Autodesk Inventor part; units mm, degrees
ref_plane "Work Plane1" through (29, 0, 0) normal (0, -1, 0) x (1, 0, 0)
ref_plane "YZ Plane" through (0, 0, 0) normal (1, 0, 0) x (0, 1, 0)
ref_plane "XZ Plane" through (0, 0, 0) normal (0, 1, 0) x (-1, 0, 0)
sketch "Sketch1" plane through (0, 0, 0) normal (0, 0, 1) x (1, 0, 0)
  line L0 (-1, 0) -> (16, 0)
  line L1 (16, 0) -> (16, 2)
  line L2 (16, 2) -> (2, 2)
  line L3 (2, 2) -> (1.5705, 2)
  line L4 (1.5705, 2) -> (0, 2)
  line L5 (0, 2) -> (0, 3.5)
  line L6 (0, 3.5) -> (-4, 3.5)
  line L7 (-4, 3.5) -> (-4, 1.7321)
  line L8 (-4, 1.7321) -> (-2, 1.7321)
  line L9 (-2, 1.7321) -> (-1, 0)
  line L10 (-8, 0) -> (20, 0)
  line L11 (0, -0.7) -> (0, 4.2)
  line L12 (2, 2) -> (0, 2) construction
  dimension "d1" = 14
  dimension "d2" = 0.4295
  dimension "d3" = 4
  dimension "d4" = 2
  dimension "d5" = 60
  dimension "d6" = 4
  dimension "d7" = 4
  dimension "d8" = 3.4641
  dimension "d9" = 7
  dimension "d26" = 16
revolve "Body" add sketch "Sketch1" angle 360 about axis through (-1, 0, 0) along (1, 0, 0)
sketch "Sketch2" plane through (-4, 0, 0) normal (-1, 0, 0) x (0, 0, 1)
  circle A0 centre (0, 0) radius 1.7321
  line L0 (0, -4.9) -> (0, 4.9)
  line L1 (-4.9, 0) -> (4.9, 0)
  line L2 (1.7321, 0) -> (0.866, -1.5)
  line L3 (0.866, -1.5) -> (-0.866, -1.5)
  line L4 (-0.866, -1.5) -> (-1.7321, 0)
  line L5 (-1.7321, 0) -> (-0.866, 1.5)
  line L6 (-0.866, 1.5) -> (0.866, 1.5)
  line L7 (0.866, 1.5) -> (1.7321, 0)
extrude "Slot" add sketch "Sketch2" against normal up to next contours L7 A0 | A0 L2 | L6 L0 A0 | A0 L0 L3 | L0 L6 A0 | A0 L3 L0 | L4 A0 | A0 L5
fillet "Fillet1" radius 0.4 1 edges at (-4, -3.5, 0)
thread "Thread"
chamfer "Chamfer1" distance 0.4294 distance2 0.4294 1 edges at (16, -2, 0) measured on face at (16, 0.527, -0.2661)
ref_plane "Work Plane1" through (29, 0, 0) normal (0, -1, 0) x (1, 0, 0)
fillet "Fillet2" radius 0.1 1 edges at (0, -2, 0)
equation "\"d1\" = GEL"
equation "\"d3\" = KOH"
equation "\"d4\" = INTI"
equation "\"d6\" = GD"
equation "\"d7\" = BDM"
equation "\"d8\" = 1.1547 * SW"
equation "\"d9\" = KOD"
equation "\"d26\" = NLG"
equation "\"d30\" = R"
equation "\"d17\" = RR"
equation "\"d13\" = GEL"
equation "\"d15\" = -0.5 * SPD + 0.5 * GD"
equation "\"d16\" = GUL"
equation "\"GD\" = NND"
equation "\"NLG\" = 16"
equation "\"GEL\" = 14"
equation "\"KOD\" = 7"
equation "\"KOH\" = NND"
equation "\"INTI\" = 2"
equation "\"GAL\" = 0.61345 * PTC"
equation "\"GUL\" = 0.61345 * PTC"
equation "\"BDM\" = NND"
equation "\"SW\" = 3"
equation "\"RR\" = 0.1 * NND"
equation "\"SPD\" = NND - 1.2269 * PTC"
equation "\"R\" = 0.1"
equation "\"PHH\" = 0.13"
equation "\"GD1\" = THREADDIA - 1.2269 * PTC"
equation "\"THREADDIA\" = 4"
equation "\"FAWI\" = 45deg"
equation "\"PTC\" = 0.7"
equation "\"KOH1\" = 3.6"
equation "\"NND\" = 4"
equation "\"TOA\" = 30deg"
equation "\"E0\" = 1.155 * SW"
properties part number "AS 1420 - 1973 - M4 x 16" material "Steel, Mild"
Design review of the part built by this model. Coordinates are the model's own, in mm. A direction names the side the tool comes from. Coordinates: 2 decimals unless noted, no trailing zeros. Loops run counter-clockwise (first coordinate to the right, second up) from the corner with the lowest first, then second, coordinate; pieces in that order, holes last. Notation, with made-up numbers: (-1.75, 32) -> (45.25, 32) arc R17 ccw to (45.25, 60) -> close; hole circle Ø5 at (44, -27). An arc over 180 degrees is marked (long way). Use a Markdown table: item, result. Add a question column.
Item 1: The part is to be moulded in two halves that separate along Z. For faces 4 (the cylindrical face through (-1.825, 3.233, 1.341)), 5 (the flat face through (16, 0, 0)), 6 (the conical face through (-1, 0, 0)), say which applies: +Z half, -Z half, draft (parallel to the pull), parting line (faces both ways), or undercut.
Item 2: Wall thickness on L1, parallel to X at y = 0.75, z = -2.75; L2, parallel to Y at x = -2.25, z = 1; L3, parallel to Y at x = 13.5, z = -1.75: over which ranges is each line inside the solid? List them lowest first. Write a range as from..to.
Item 3: Clearance check with flat-ended pins moving along their axes: P1, Ø1.5, axis at x = 5.5, z = 1, coming from the -Y side; P2, Ø1.5, axis at y = 1.5, z = -2.5, coming from the +X side; P3, Ø1, axis at x = 11.5, y = -1, coming from the +Z side. State where each tip first meets the part, or that it passes through.
Item 4: Machinability: for faces 1 (the flat face through (-2.948, 0.74, -1.305)), 2 (the cylindrical face through (8, 0, 2)), 3 (the flat face through (-4, -1.3, 1.3)), which of the approach directions +Z, -Z, +X, -X, +Y, -Y give a long, thin tool a straight path to every point of the face, cutting with its end or side? Answer none if there is none.
Item 5: We need section A-A, the plane x = 12.5. Write out the cut boundary in (y, z).
Numbers:
| question | item | result |
|---|---|---|
| 1 | face 4 | parting line |
| 1 | face 5 | draft |
| 1 | face 6 | undercut |
| 2 | L1 | x = -4..0 |
| 2 | L2 | y = -3.35..-1.27, 1.27..3.35 |
| 2 | L3 | y = -0.97..0.97 |
| 3 | P1 | stops at y = -1.98 |
| 3 | P2 | stops at x = 0 |
| 3 | P3 | stops at z = 1.94 |
| 4 | face 1 | -X |
| 4 | face 2 | +X |
| 4 | face 3 | +Z, -Z, -X, +Y, -Y |
| 5 | outline | circle Ø4 at (0, 0) |
